Can you work these out from the model? Positions are in its coordinate system, mm. A direction names the side the tool comes from. Give positions to 0.01 mm unless a question says otherwise; leave off trailing zeros. Order: outer loops, then holes, each group sorted by start corner. A loop starts at its lowest first (then second) coordinate and runs counter-clockwise, first axis right, second up. Notation, with made-up numbers: M 89.25,20.25 L 108.25,20.25 A16 cw 108.25,30.25 Z; hole C -10,9 d5. An arc over 180 degrees is marked long. Answer as a JSON object with one key per item and string values.
```python
from build123d import *

# Parameters (mm, degrees)
SKETCH1_W             = 140
SKETCH1_H             = 87.5
BOSS_EXTRUDE1_DEPTH   = 10
SKETCH2_W             = 90
SKETCH2_H             = 81
CUT_EXTRUDE1_DEPTH    = 4.25
SKETCH5_W             = 23
SKETCH5_H             = 80
CUT_EXTRUDE2_DEPTH    = 8
F_6_CLEARANCE_HOLE1_D = 3.7973
CUT_EXTRUDE4_DEPTH    = 3
FILLET1_R             = 7.5
SKETCH15_R            = 4.55
CUT_EXTRUDE3_DEPTH    = 7.5
FILLET2_R             = 1
FILLET3_R             = 5


with BuildPart() as part:
    # Sketch1 → Boss-Extrude1 (new body)
    with BuildSketch(Plane(origin=(0, 0, 0), x_dir=(1, 0, 0), z_dir=(0, 1, 0))):
        with Locations((70, 43.75)):
            Rectangle(SKETCH1_W, SKETCH1_H)
    extrude(amount=BOSS_EXTRUDE1_DEPTH)

    # Sketch2 → Cut-Extrude1 (cut)
    with BuildSketch(Plane(origin=(0, 10, 0), x_dir=(1, 0, 0), z_dir=(0, 1, 0))):
        with Locations((90.5, 43.75)):
            Rectangle(SKETCH2_W, SKETCH2_H)
    extrude(amount=-CUT_EXTRUDE1_DEPTH, mode=Mode.SUBTRACT)

    # Sketch5 → Cut-Extrude2 (cut)
    with BuildSketch(Plane(origin=(0, 10, 0), x_dir=(1, 0, 0), z_dir=(0, 1, 0))):
        with Locations((14.5, 43.75)):
            Rectangle(SKETCH5_W, SKETCH5_H)
    extrude(amount=-CUT_EXTRUDE2_DEPTH, mode=Mode.SUBTRACT)

    # #6 Clearance Hole1 (through all)
    with Locations(Plane(origin=(0, 5.75, 0), x_dir=(1, 0, 0), z_dir=(0, 1, 0))):
        with Locations((56.75, 47.25), (93.25, 76.25), (113.25, 35.75)):
            Hole(F_6_CLEARANCE_HOLE1_D / 2)

    # Sketch19 → Cut-Extrude4 (cut)
    with BuildSketch(Plane(origin=(0, 5.75, 0), x_dir=(1, 0, 0), z_dir=(0, 1, 0))):
        Polygon((59.059401077, 51.25), (54.440598923, 51.25), (52.131197846, 47.25), (54.440598923, 43.25), (59.059401077, 43.25), (61.368802154, 47.25), align=None)
        Polygon((97.868802154, 76.25), (95.559401077, 80.25), (90.940598923, 80.25), (88.631197846, 76.25), (90.940598923, 72.25), (95.559401077, 72.25), align=None)
        Polygon((117.868802154, 35.75), (115.559401077, 39.75), (110.940598923, 39.75), (108.631197846, 35.75), (110.940598923, 31.75), (115.559401077, 31.75), align=None)
    extrude(amount=-CUT_EXTRUDE4_DEPTH, mode=Mode.SUBTRACT)

    # Fillet1
    fillet1_edges = [part.edges().sort_by_distance(p)[0] for p in [
        (0, 5, -87.5),
        (140, 5, -87.5),
        (140, 5, 0),
        (0, 5, 0),
    ]]
    fillet(fillet1_edges, radius=FILLET1_R)

    # Sketch15 → Cut-Extrude3 (cut)
    with BuildSketch(Plane(origin=(0, 10, 0), x_dir=(1, 0, 0), z_dir=(0, 1, 0))):
        with Locations(Location((35.75, 43.75, 0), (0, 0, 270))):
            Circle(SKETCH15_R)
        with Locations(Location((35.75, 58.75, 0), (0, 0, 270))):
            Circle(SKETCH15_R)
        with Locations(Location((35.75, 28.75, 0), (0, 0, 270))):
            Circle(SKETCH15_R)
    extrude(amount=-CUT_EXTRUDE3_DEPTH, mode=Mode.SUBTRACT)

    # Fillet2
    fillet2_edges = [part.edges().sort_by_distance(p)[0] for p in [
        (45.5, 7.875, -3.25),
        (45.5, 7.875, -84.25),
        (135.5, 7.875, -84.25),
        (135.5, 7.875, -3.25),
        (3, 6, -3.75),
        (3, 6, -83.75),
        (26, 6, -83.75),
        (26, 6, -3.75),
    ]]
    fillet(fillet2_edges, radius=FILLET2_R)

    # Fillet3
    fillet3_edges = [part.edges().sort_by_distance(p)[0] for p in [
        (70, 0, 0),
        (0, 0, -43.75),
        (70, 0, -87.5),
        (140, 0, -43.75),
        (137.803300859, 0, -2.196699141),
        (137.803300859, 0, -85.303300859),
        (2.196699141, 0, -85.303300859),
        (2.196699141, 0, -2.196699141),
    ]]
    fillet(fillet3_edges, radius=FILLET3_R)


solid = part.part
```
1) I want a section at A-A on y = 8.5. Write out the boundary of the cut face in (x, z), and give its area (3 significant figures).
Results found:
{"outline": "M 0,-80 A7.5 ccw 7.5,-87.5 L 132.5,-87.5 A7.5 ccw 140,-80 L 140,-7.5 A7.5 ccw 132.5,0 L 7.5,0 A7.5 ccw 0,-7.5 Z; hole M 3,-82.75 A1 ccw 4,-83.75 L 25,-83.75 A1 ccw 26,-82.75 L 26,-4.75 A1 ccw 25,-3.75 L 4,-3.75 A1 ccw 3,-4.75 Z; hole C 35.75,-58.75 d9.1; hole C 35.75,-43.75 d9.1; hole C 35.75,-28.75 d9.1; hole M 45.5,-83.25 A1 ccw 46.5,-84.25 L 134.5,-84.25 A1 ccw 135.5,-83.25 L 135.5,-4.25 A1 ccw 134.5,-3.25 L 46.5,-3.25 A1 ccw 45.5,-4.25 Z", "area": "2,880 mm²"}
2) I'm going to push flat-ended pins straight in: pin 1 Ø8 at (x, z) = (109, -66) entering from +Y; pin 2 Ø4 at (x, z) = (113, -36.5) entering from +Y; pin 3 Ø3.5 at (x, z) = (93.25, -76.25) entering from +Y; pin 4 Ø8 at (x, z) = (35.75, -58.75) entering from +Y. Where does each tip first touch, or does it pass through?
Results found:
{"pin 1": "stops at y = 5.75", "pin 2": "stops at y = 2.75", "pin 3": "passes through", "pin 4": "stops at y = 2.5"}
3) I need wall thicknesses on L1, parallel to X at y = 6.75, z = -16; L2, parallel to X at y = 7.25, z = -58.75; L3, parallel to X at y = 5.25, z = -28.75. Which ranges of each line are inside material? Lowest first, please.
Results found:
{"L1": "x = 0 to 3, 26 to 45.5, 135.5 to 140", "L2": "x = 0 to 3, 26 to 31.2, 40.3 to 45.5, 135.5 to 140", "L3": "x = 0 to 3, 26 to 31.2, 40.3 to 140"}
4) For faces 4 (the face through (113, 4, -39.75)), 5 (the face through (113.497, 1.356, -37.632)), which set-ups out of +Z, -Z, +X, -X, +Y, -Y let a thin tool reach every point of the face, with its end or its side?
Results found:
{"face 4": "+Y", "face 5": "+Y, -Y"}
5) I want a section at B-B on x = 56.75. Write out the boundary of the cut face in (y, z).
Results found:
{"outline": "M 0,-82.5 A5 ccw 5,-87.5 L 10,-87.5 L 10,-84.25 L 5.75,-84.25 L 5.75,-51.25 L 2.75,-51.25 L 2.75,-49.15 L 0,-49.15 Z; M 0,-45.35 L 2.75,-45.35 L 2.75,-43.25 L 5.75,-43.25 L 5.75,-3.25 L 10,-3.25 L 10,0 L 5,0 A5 ccw 0,-5 Z"}
6) Thinking about a two-plate mould opening in Z: for faces 1 (the face through (137.745, 7.535, -85.361)), 2 (the face through (14, 6, -83.75)), 3 (the face through (139, 2, -44)), which applies, pulls with the +Z half, pulls with the -Z half, needs draft (parallel to the pull), parting line crosses it, or undercut?
Results found:
{"face 1": "pulls with the -Z half", "face 2": "undercut", "face 3": "needs draft"}
7) I want a section at D-D on x = 20. Write out the boundary of the cut face in (y, z).
Results found:
{"outline": "M 0,-82.5 A5 ccw 5,-87.5 L 10,-87.5 L 10,-83.75 L 2,-83.75 L 2,-3.75 L 10,-3.75 L 10,0 L 5,0 A5 ccw 0,-5 Z"}
8) I want a section at C-C on z = -58.75. Write out the boundary of the cut face in (x, y).
Results found:
{"outline": "M 0,5 A5 ccw 5,0 L 135,0 A5 ccw 140,5 L 140,10 L 135.5,10 L 135.5,5.75 L 45.5,5.75 L 45.5,10 L 40.3,10 L 40.3,2.5 L 31.2,2.5 L 31.2,10 L 26,10 L 26,2 L 3,2 L 3,10 L 0,10 Z"}
